```python
from build123d import *

# Parameters (mm, degrees)
BOSS_EXTRUDE1_DEPTH = 16
CUT_EXTRUDE1_DEPTH  = 12
SKETCH4_W           = 72
SKETCH4_H           = 5
CUT_EXTRUDE2_DEPTH  = 16
SKETCH5_R           = 35
CUT_EXTRUDE3_DEPTH  = 16
CUT_EXTRUDE4_DEPTH  = 10
SKETCH7_R           = 42
BOSS_EXTRUDE2_DEPTH = 5
SKETCH8_R           = 3.5
SKETCH8_R_2         = 1.5
BOSS_EXTRUDE3_DEPTH = 12
SKETCH9_R           = 1.5
CUT_EXTRUDE5_DEPTH  = 12


with BuildPart() as part:
    # Sketch1 → Boss-Extrude1 (new body)
    with BuildSketch(Plane(origin=(0, 0, 0), x_dir=(1, 0, 0), z_dir=(0, 1, 0))):
        with BuildLine():
            Line((24.684271836, -45.0001724), (24.684271836, 44.9998276))
            Line((24.684271836, 44.9998276), (31.307293766, 44.9998276))
            ThreePointArc((31.307293766, 44.9998276), (-55.315728163, 0.000299848), (31.306803106, -45.0001724))
            Line((31.306803106, -45.0001724), (24.684271836, -45.0001724))
        make_face()
        with BuildLine():
            Line((31.307293766, 44.9998276), (24.684271836, 44.9998276))
            Line((24.684271836, 44.9998276), (24.684271836, -45.0001724))
            Line((24.684271836, -45.0001724), (31.306803106, -45.0001724))
            ThreePointArc((31.306803106, -45.0001724), (48.491234556, -25.355086079), (54.684271836, 0))
            ThreePointArc((54.684271836, 0), (48.491372785, 25.354819994), (31.307293766, 44.9998276))
        make_face()
        with BuildLine():
            Line((55.315728164, 44.9998276), (31.307293766, 44.9998276))
            ThreePointArc((31.307293766, 44.9998276), (48.491372785, 25.354819994), (54.684271836, 0))
            ThreePointArc((54.684271836, 0), (48.491234556, -25.355086079), (31.306803106, -45.0001724))
            Line((31.306803106, -45.0001724), (55.315728164, -45.0001724))
            Line((55.315728164, -45.0001724), (55.315728164, 44.9998276))
        make_face()
    extrude(amount=BOSS_EXTRUDE1_DEPTH)

    # Sketch3 → Cut-Extrude1 (cut)
    with BuildSketch(Plane.XZ):
        with BuildLine():
            ThreePointArc((50, 0), (44.646173327, 22.510424413), (29.73123171, 40.2001724))
            Line((29.73123171, 40.2001724), (13.648760289, 40.2001724))
            Line((13.648760289, 40.2001724), (13.648760289, -40.1998276))
            Line((13.648760289, -40.1998276), (29.731697916, -40.1998276))
            ThreePointArc((29.731697916, -40.1998276), (44.646303855, -22.510165528), (50, 0))
        make_face()
        with BuildLine():
            Line((13.648760289, 40.2001724), (29.73123171, 40.2001724))
            ThreePointArc((29.73123171, 40.2001724), (-49.999999999, -0.000289929), (29.731697916, -40.1998276))
            Line((29.731697916, -40.1998276), (13.648760289, -40.1998276))
            Line((13.648760289, -40.1998276), (13.648760289, 40.2001724))
        make_face()
        with BuildLine():
            Line((50.315728164, -40.1998276), (50.315728164, 40.2001724))
            Line((50.315728164, 40.2001724), (29.73123171, 40.2001724))
            ThreePointArc((29.73123171, 40.2001724), (44.646173327, 22.510424413), (50, 0))
            ThreePointArc((50, 0), (44.646303855, -22.510165528), (29.731697916, -40.1998276))
            Line((29.731697916, -40.1998276), (50.315728164, -40.1998276))
        make_face()
    extrude(amount=-CUT_EXTRUDE1_DEPTH, mode=Mode.SUBTRACT)

    # Sketch4 → Cut-Extrude2 (cut)
    with BuildSketch(Plane(origin=(55.315728164, 0, 0), x_dir=(0, 0, -1), z_dir=(1, 0, 0))):
        with Locations((-0.0001724, 2.5)):
            Rectangle(SKETCH4_W, SKETCH4_H)
    extrude(amount=-CUT_EXTRUDE2_DEPTH, mode=Mode.SUBTRACT)

    # Sketch5 → Cut-Extrude3 (cut)
    with BuildSketch(Plane(origin=(0, 16, 0), x_dir=(1, 0, 0), z_dir=(0, 1, 0))):
        Circle(SKETCH5_R)
    extrude(amount=-CUT_EXTRUDE3_DEPTH, mode=Mode.SUBTRACT)

    # Sketch6 → Cut-Extrude4 (cut)
    with BuildSketch(Plane(origin=(0, 16, 0), x_dir=(1, 0, 0), z_dir=(0, 1, 0))):
        with BuildLine():
            Line((-28.284271247, -28.284271247), (-24.748737342, -24.748737342))
            ThreePointArc((-24.748737342, -24.748737342), (-27.76736691, -21.306650015), (-30.310889132, -17.5))
            Line((-30.310889132, -17.5), (-34.641016151, -20))
            ThreePointArc((-34.641016151, -20), (-31.734133612, -24.35045716), (-28.284271247, -28.284271247))
        make_face()
        with BuildLine():
            Line((-34.641016151, -20), (-30.310889132, -17.5))
            ThreePointArc((-30.310889132, -17.5), (-32.335783638, -13.393920133), (-33.80740392, -9.058666579))
            Line((-33.80740392, -9.058666579), (-38.637033052, -10.352761804))
            ThreePointArc((-38.637033052, -10.352761804), (-36.9551813, -15.307337295), (-34.641016151, -20))
        make_face()
        with BuildLine():
            Line((-10.352761804, 38.637033052), (-9.058666579, 33.80740392))
            ThreePointArc((-9.058666579, 33.80740392), (0, 35), (9.058666579, 33.80740392))
            Line((9.058666579, 33.80740392), (10.352761804, 38.637033052))
            ThreePointArc((10.352761804, 38.637033052), (0, 40), (-10.352761804, 38.637033052))
        make_face()
        with BuildLine():
            ThreePointArc((33.831018509, -8.970071717), (32.370760151, -13.309165535), (30.356629112, -17.420535841))
            Line((30.356629112, -17.420535841), (34.693290413, -19.909183818))
            ThreePointArc((34.693290413, -19.909183818), (36.995154458, -15.210474897), (38.664021154, -10.251510534))
            Line((38.664021154, -10.251510534), (33.831018509, -8.970071717))
        make_face()
        with BuildLine():
            ThreePointArc((30.356629112, -17.420535841), (27.823087732, -21.233835948), (24.813485607, -24.683819236))
            Line((24.813485607, -24.683819236), (28.358269265, -28.210079126))
            ThreePointArc((28.358269265, -28.210079126), (31.79781455, -24.267241084), (34.693290413, -19.909183818))
            Line((34.693290413, -19.909183818), (30.356629112, -17.420535841))
        make_face()
    extrude(amount=-CUT_EXTRUDE4_DEPTH, mode=Mode.SUBTRACT)

    # Sketch7 → Boss-Extrude2 (add)
    with BuildSketch(Plane.XZ.offset(-12)):
        Circle(SKETCH7_R)
        with BuildLine():
            ThreePointArc((-28.284271247, 28.284271247), (-10.352761804, 38.637033052), (10.352761804, 38.637033052))
            Line((10.352761804, 38.637033052), (9.058666579, 33.80740392))
            ThreePointArc((9.058666579, 33.80740392), (10.524702983, 33.380093276), (11.970705016, 32.889241728))
            Line((11.970705016, 32.889241728), (13.680805733, 37.587704831))
            ThreePointArc((13.680805733, 37.587704831), (21.53615385, 33.707478063), (28.358269265, 28.210079126))
            ThreePointArc((28.358269265, 28.210079126), (34.693290413, 19.909183818), (38.664021154, 10.251510534))
            ThreePointArc((38.664021154, 10.251510534), (38.623439557, -10.40336084), (28.284271247, -28.284271247))
            Line((28.284271247, -28.284271247), (24.748737342, -24.748737342))
            ThreePointArc((24.748737342, -24.748737342), (23.645657267, -25.804706788), (22.497566339, -26.811555509))
            Line((22.497566339, -26.811555509), (25.711504387, -30.641777725))
            ThreePointArc((25.711504387, -30.641777725), (18.469944529, -35.480433327), (10.352761804, -38.637033052))
            ThreePointArc((10.352761804, -38.637033052), (0, -40), (-10.352761804, -38.637033052))
            ThreePointArc((-10.352761804, -38.637033052), (-28.284271247, -28.284271247), (-38.637033052, -10.352761804))
            Line((-38.637033052, -10.352761804), (-33.80740392, -9.058666579))
            ThreePointArc((-33.80740392, -9.058666579), (-34.170360249, -7.575386488), (-34.468271355, -6.077686218))
            Line((-34.468271355, -6.077686218), (-39.39231012, -6.945927107))
            ThreePointArc((-39.39231012, -6.945927107), (-39.961928863, 1.744775495), (-38.637033052, 10.352761804))
            ThreePointArc((-38.637033052, 10.352761804), (-34.641016151, 20), (-28.284271247, 28.284271247))
        make_face(mode=Mode.SUBTRACT)
    extrude(amount=BOSS_EXTRUDE2_DEPTH)

    # Sketch8 → Boss-Extrude3 (add)
    with BuildSketch(Plane.XZ.offset(-12)):
        with Locations((-25, 43.301270189)):
            Circle(SKETCH8_R)
        with Locations((-25, 43.301270189)):
            Circle(SKETCH8_R_2, mode=Mode.SUBTRACT)
        with Locations((-25, -43.301270189)):
            Circle(SKETCH8_R)
        with Locations((-25, -43.301270189)):
            Circle(SKETCH8_R_2, mode=Mode.SUBTRACT)
        with Locations((31.306803106, 40.2001724)):
            Circle(SKETCH8_R)
        with Locations((31.306803106, 40.2001724)):
            Circle(SKETCH8_R_2, mode=Mode.SUBTRACT)
        with Locations((31.307293766, -40.1998276)):
            Circle(SKETCH8_R)
        with Locations((31.307293766, -40.1998276)):
            Circle(SKETCH8_R_2, mode=Mode.SUBTRACT)
    extrude(amount=BOSS_EXTRUDE3_DEPTH)

    # Sketch9 → Cut-Extrude5 (cut)
    with BuildSketch(Plane.XZ.offset(-12)):
        with Locations((-25, 43.301270189)):
            Circle(SKETCH9_R)
        with Locations((31.306803106, 40.2001724)):
            Circle(SKETCH9_R)
        with Locations((-25, -43.301270189)):
            Circle(SKETCH9_R)
        with Locations((31.307293766, -40.1998276)):
            Circle(SKETCH9_R)
    extrude(amount=CUT_EXTRUDE5_DEPTH, mode=Mode.SUBTRACT)


solid = part.part
```
Read the model definition and answer for the solid it produces. Units are mm, in the model's axes. A direction names the side the tool comes from. Coordinates: 2 decimals unless noted, no trailing zeros. Loops run counter-clockwise (first coordinate to the right, second up) from the corner with the lowest first, then second, coordinate; pieces in that order, holes last. Notation, with made-up numbers: (-30.5, 84.25) -> (7.5, 84.25) arc R25 ccw to (7.5, 103.25) -> close; hole circle Ø2 at (27.25, -40). An arc over 180 degrees is marked (long way). Return JSON: item names as keys, results as strings.
Item 1: Find the intervals of material crossed by probe 1 along X at (y, z) = (3.25, 37); probe 2 along X at (y, z) = (9.75, -11) (1 decimal); probe 3 along X at (y, z) = (10.25, -3), in increasing order.
Answers:
{"probe 1": "x = -41.01 to -33.63, 29.89 to 32.72, 50.32 to 55.32", "probe 2": "x = -54.2 to -48.8, -40.5 to -38.5, 38.5 to 40.5, 50.3 to 55.3", "probe 3": "x = -55.23 to -49.91, -41.89 to -39.89, 39.89 to 41.89, 50.32 to 55.32"}
Item 2: Flat-ended cylindrical pins translate along their axes: P1, Ø1.5, axis at x = -25, z = -44, coming from the -Y side; P2, Ø1, axis at y = 9.5, z = -21.5, coming from the -X side; P3, Ø1.5, axis at x = -15.5, y = 13, coming from the +Z side. Find the tip coordinate at first contact, or state that the pin passes through.
Answers:
{"P1": "stops at y = 12", "P2": "stops at x = -51.15", "P3": "stops at z = 53.07"}
Item 3: For a pull along X with two mould halves and no side action, classify faces 4 (the flat face through (42, 6, -40.2)), 5 (the cylindrical face through (30.78, 6.08, -36.74)), 6 (the flat face through (36, 16, -1)) as +X half, -X half, draft (parallel to the pull), parting line (faces both ways), or undercut.
Answers:
{"face 4": "undercut", "face 5": "undercut", "face 6": "draft"}
Item 4: Find section A-A (z = 0). Determine the outline of the cut face in (x, y).
Answers:
{"outline": "(-55.32, 0) -> (-50, 0) -> (-50, 12) -> (-42, 12) -> (-42, 7) -> (-40, 7) -> (-40, 12) -> (-35, 12) -> (-35, 16) -> (-55.32, 16) -> close; (35, 12) -> (40, 12) -> (40, 7) -> (42, 7) -> (42, 12) -> (50.32, 12) -> (50.32, 5) -> (55.32, 5) -> (55.32, 16) -> (35, 16) -> close"}
Item 5: For faces 1 (the flat face through (-9.715, 14.028, -36.256)), 2 (the flat face through (43, 8, -45)), 3 (the cylindrical face through (30.61, 6.08, 36.77)), determine the directions among +Z, -Z, +X, -X, +Y, -Y from which every point of the face is accessible in a straight line to the end or side of a thin tool.
Answers:
{"face 1": "+Y, -Y", "face 2": "-Z, +X, +Y, -Y", "face 3": "-Y"}
Item 6: Find section D-D (z = 48). Determine the outline of the cut face in (x, y).
Answers:
{"outline": "(-27.17, 0) -> (-14, 0) -> (-14, 12) -> (14, 12) -> (14, 0) -> (26.54, 0) -> (26.54, 16) -> (-27.17, 16) -> close"}
Item 7: Find section B-B (y = 14.25). Determine the outline of the cut face in (x, z).
Answers:
{"outline": "(31.31, -45) -> (55.32, -45) -> (55.32, 45) -> (31.31, 45) arc R55 ccw (long way) to start; hole (-38.64, 10.35) -> (-33.81, 9.06) arc R35 ccw to (-9.06, -33.81) -> (-10.35, -38.64) arc R40 ccw to (10.35, -38.64) -> (9.06, -33.81) arc R35 ccw to (33.83, 8.97) -> (38.66, 10.25) arc R40 ccw to (28.36, 28.21) -> (24.81, 24.68) arc R35 ccw to (-24.75, 24.75) -> (-28.28, 28.28) arc R40 ccw to start"}
Item 8: Find section C-C (x = 0). Determine the outline of the cut face in (y, z).
Answers:
{"outline": "(0, -55) -> (16, -55) -> (16, -40) -> (7, -40) -> (7, -42) -> (12, -42) -> (12, -50) -> (0, -50) -> close; (0, 50) -> (12, 50) -> (12, 42) -> (7, 42) -> (7, 40) -> (12, 40) -> (12, 35) -> (16, 35) -> (16, 55) -> (0, 55) -> close"}
